Check sheet for the modelled part. Datum: model origin and axes. Units: mm. Face numbers are marked on the shaded views. Give positions to 0.01 mm unless a question says otherwise; leave off trailing zeros. Loops run counter-clockwise (first coordinate to the right, second up) from the corner with the lowest first, then second, coordinate; pieces in that order, holes last. Notation, with made-up numbers: (63, 73) - (114, 73) arc R18 ccw to (114, 96) - close; hole circle Ø1 at (-39, -39). An arc over 180 degrees is marked (long way). Answer in a Markdown table with one row per item. Add a question column.
(1) Draft check along X on the marked faces 1, 2 and 3. Enter one of: released by +X, released by -X, zero draft, split by the parting line, or undercut.
(2) Thickness scan on L1, parallel to Y at x = -0.75, z = -3.25; L2, parallel to Z at x = -1, y = -1.7; L3, parallel to Y at x = 0.25, z = -2. Record the ranges inside material, lowest first.
(3) Go/stop test with flat-tipped pins: P1, Ø0.7, axis at x = -0.5, z = -0.5, coming from the +Y side; P2, Ø4, axis at x = -3, z = -3, coming from the +Y side. Record where each tip stops, or that it passes through.
(4) Sectioned sample at C-C on y = -1.65. Enter the section's corners in (x, z).
from build123d import *

# Parameters (mm, degrees)
F1_DEPTH     = 3
F2_SIZE2     = 1.49999
F2_SIZE      = 1.49999
F3_W         = 1.7351090792
F3_H         = 1.7351090792
F4_DEPTH     = 0.45
F5_T4_DEPTH  = 3.4702181583
F5_T9_DEPTH  = 3.4702181583
F5_T14_DEPTH = 3.4702181583
F5_T19_DEPTH = 3.4702181583
F6_T1_DEPTH  = 16.5056825173
F6_T3_DEPTH  = 16.5056825173


# Not quite as in the source:
# - a fillet or chamfer that OpenCascade refuses, or shapes differently, is made with other operations: its cross-section is extruded or revolved along the edge and cut away or added
# - a fillet or chamfer is up to 0.001 mm smaller than in the source, because OpenCascade refuses the exact size


with BuildPart() as f1:
    # F0 (on Front) → F1 (new body)
    with BuildSketch(Plane.XZ):
        Polygon((4.575161729, 4.575161729), (0, 4.575161729), (-4.575161729, 4.575161729), (-4.575161729, 0), (-4.575161729, -4.575161729), (0, -4.575161729), (4.575161729, -4.575161729), (4.575161729, 0), align=None)
    extrude(amount=F1_DEPTH)

    # F2 (size 1.5 and 1.5 in the source; OpenCascade refuses exactly that, so slightly less here)
    f2_edges = [f1.edges().sort_by_distance(p)[0] for p in [
        (0, -3, 4.575162),
        (-4.575162, -3, 0),
        (0, -3, -4.575162),
        (4.575162, -3, 0),
        (0, 0, 4.575162),
        (-4.575162, 0, 0),
        (0, 0, -4.575162),
        (4.575162, 0, 0),
    ]]
    chamfer(f2_edges, length=F2_SIZE, length2=F2_SIZE2)

    # F3 (on face) → F4 (cut)
    with BuildSketch(Plane(origin=(0, 0, 0), x_dir=(-1, 0, 0), z_dir=(0, 1, 0))):
        Polygon((0, 1.7351090792), (0, 0), (-1.7351090792, 0), (-1.7351090792, -1.7351090792), (0, -1.7351090792), (1.7351090792, -1.7351090792), (1.7351090792, 0), (1.7351090792, 1.7351090792), align=None)
        with Locations((-0.8675545396, 0.8675545396)):
            Rectangle(F3_W, F3_H)
    extrude(amount=-F4_DEPTH, mode=Mode.SUBTRACT)

    # F5: chamfer of 0.6 on 4 edges, made by hand


with BuildPart() as f5_tool2:
    # F5_s3 → F5_t4 (new body)
    with BuildSketch(Plane.YZ.offset(-1.7351090792)):
        Polygon((0.15, 1.7351090792), (-0.45, 1.1351090792), (-0.45, 1.7351090792), align=None)
    extrude(amount=F5_T4_DEPTH)

    split(bisect_by=Plane.XZ, keep=Keep.TOP)


with BuildPart() as f1_1:
    add(f1.part)

    # F5_t1: union F5_tool2
    add(f5_tool2.part)


with BuildPart() as f5_tool7:
    # F5_s8 → F5_t9 (new body)
    with BuildSketch(Plane.XY.offset(1.7351090792)):
        Polygon((1.7351090792, 0.15), (1.1351090792, -0.45), (1.7351090792, -0.45), align=None)
    extrude(amount=-F5_T9_DEPTH)

    split(bisect_by=Plane.XZ, keep=Keep.TOP)


with BuildPart() as f1_2:
    add(f1_1.part)

    # F5_t6: union F5_tool7
    add(f5_tool7.part)


with BuildPart() as f5_tool12:
    # F5_s13 → F5_t14 (new body)
    with BuildSketch(Plane.YZ.offset(1.7351090792)):
        Polygon((0.15, -1.7351090792), (-0.45, -1.1351090792), (-0.45, -1.7351090792), align=None)
    extrude(amount=-F5_T14_DEPTH)

    split(bisect_by=Plane.XZ, keep=Keep.TOP)


with BuildPart() as f1_3:
    add(f1_2.part)

    # F5_t11: union F5_tool12
    add(f5_tool12.part)


with BuildPart() as f5_tool17:
    # F5_s18 → F5_t19 (new body)
    with BuildSketch(Plane.XY.offset(-1.7351090792)):
        Polygon((-1.7351090792, 0.15), (-1.1351090792, -0.45), (-1.7351090792, -0.45), align=None)
    extrude(amount=F5_T19_DEPTH)

    split(bisect_by=Plane.XZ, keep=Keep.TOP)


with BuildPart() as f1_4:
    add(f1_3.part)

    # F5_t16: union F5_tool17
    add(f5_tool17.part)

    # F6: fillet of radius 5 on 4 edges, made by hand

    # F6_s2 → F6_t1 (cut)
    with BuildSketch(Plane.XY.offset(-8.2528412587)):
        with BuildLine():
            ThreePointArc((4.5396378231, -1.4644660941), (2.917521079, -0.3806023374), (1.0041039171, 0))
            Line((1.0041039171, 0), (3.075171729, 0))
            Line((3.075171729, 0), (4.5396378231, -1.4644660941))
        make_face()
        with BuildLine():
            ThreePointArc((-1.0041039171, 0), (-2.917521079, -0.3806023374), (-4.5396378231, -1.4644660941))
            Line((-4.5396378231, -1.4644660941), (-3.075171729, 0))
            Line((-3.075171729, 0), (-1.0041039171, 0))
        make_face()
    extrude(amount=F6_T1_DEPTH, mode=Mode.SUBTRACT)

    # F6_s4 → F6_t3 (cut)
    with BuildSketch(Plane.YZ.offset(-8.2528412587)):
        with BuildLine():
            ThreePointArc((-1.4644660941, 4.5396378231), (-0.3806023374, 2.917521079), (0, 1.0041039171))
            Line((0, 1.0041039171), (0, 3.075171729))
            Line((0, 3.075171729), (-1.4644660941, 4.5396378231))
        make_face()
        with BuildLine():
            ThreePointArc((0, -1.0041039171), (-0.3806023374, -2.917521079), (-1.4644660941, -4.5396378231))
            Line((-1.4644660941, -4.5396378231), (0, -3.075171729))
            Line((0, -3.075171729), (0, -1.0041039171))
        make_face()
    extrude(amount=F6_T3_DEPTH, mode=Mode.SUBTRACT)


solid = f1_4.part
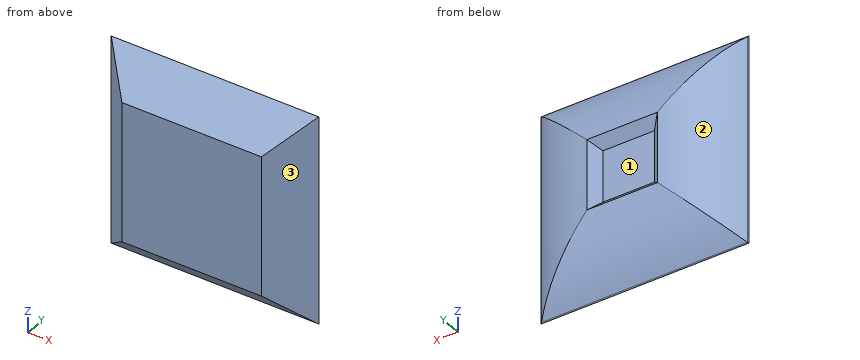
Reply:
| question | item | result |
|---|---|---|
| 1 | face 1 | undercut |
| 1 | face 2 | released by -X |
| 1 | face 3 | released by +X |
| 2 | L1 | -2.83 to -0.53 |
| 2 | L2 | -4.38 to 4.38 |
| 2 | L3 | -3 to -0.1 |
| 3 | P1 | y = -0.45 |
| 3 | P2 | y = -0.03 |
| 4 | outline | (-4.43, -4.43) - (4.43, -4.43) - (4.43, 4.43) - (-4.43, 4.43) - close |
